```python
from build123d import *

# Parameters (mm, degrees)
F0_R     = 5
F1_DEPTH = 10
F2_DEPTH = 30


with BuildPart() as f1:
    # F0 (on Front) → F1 (new body, symmetric)
    with BuildSketch(Plane.XZ):
        with BuildLine():
            Line((-25, -43.3012701892), (-5, -8.6602540378))
            ThreePointArc((-5, -8.6602540378), (-5, 8.6602540378), (10, 0))
            ThreePointArc((10, 0), (8.6602540378, -5), (5, -8.6602540378))
            Line((5, -8.6602540378), (25, -43.3012701892))
            Line((25, -43.3012701892), (10, 100))
            ThreePointArc((10, 100), (0, 90), (-10, 100))
            Line((-10, 100), (-25, -43.3012701892))
        make_face()
        with BuildLine():
            Line((47.5, -82.2724133595), (45, -77.9422863406))
            ThreePointArc((45, -77.9422863406), (41.3397459622, -81.6025403784), (40, -86.6025403784))
            Line((40, -86.6025403784), (45, -86.6025403784))
            ThreePointArc((45, -86.6025403784), (45.6698729811, -84.1025403784), (47.5, -82.2724133595))
        make_face()
        with BuildLine():
            Line((-5, -8.6602540378), (-2.5, -4.3301270189))
            ThreePointArc((-2.5, -4.3301270189), (-2.5, 4.3301270189), (5, 0))
            ThreePointArc((5, 0), (4.3301270189, -2.5), (2.5, -4.3301270189))
            Line((2.5, -4.3301270189), (5, -8.6602540378))
            ThreePointArc((5, -8.6602540378), (8.6602540378, -5), (10, 0))
            ThreePointArc((10, 0), (-5, 8.6602540378), (-5, -8.6602540378))
        make_face()
        with BuildLine():
            Line((-45, -77.9422863406), (-25, -43.3012701892))
            Line((-25, -43.3012701892), (-57.4852813742, -79.9715100853))
            ThreePointArc((-57.4852813742, -79.9715100853), (-51.6042422288, -76.7320587858), (-45, -77.9422863406))
        make_face()
        with BuildLine():
            ThreePointArc((57.4852813742, -79.9715100853), (51.6042422288, -76.7320587858), (45, -77.9422863406))
            Line((45, -77.9422863406), (47.5, -82.2724133595))
            ThreePointArc((47.5, -82.2724133595), (52.5, -82.2724133595), (55, -86.6025403784))
            ThreePointArc((55, -86.6025403784), (50, -91.6025403784), (45, -86.6025403784))
            Line((45, -86.6025403784), (40, -86.6025403784))
            ThreePointArc((40, -86.6025403784), (42.2540333076, -92.9270956988), (48, -96.4004993496))
            ThreePointArc((48, -96.4004993496), (56.3245553203, -94.3485070709), (60, -86.6025403784))
            ThreePointArc((60, -86.6025403784), (59.3502089213, -83.0566141061), (57.4852813742, -79.9715100853))
        make_face()
        with BuildLine():
            ThreePointArc((-40, -86.6025403784), (-41.3397459622, -81.6025403784), (-45, -77.9422863406))
            Line((-45, -77.9422863406), (-47.5, -82.2724133595))
            ThreePointArc((-47.5, -82.2724133595), (-45.6698729811, -84.1025403784), (-45, -86.6025403784))
            Line((-45, -86.6025403784), (-40, -86.6025403784))
        make_face()
        with BuildLine():
            Line((0, -86.6025403784), (-40, -86.6025403784))
            ThreePointArc((-40, -86.6025403784), (-42.2540333076, -92.9270956988), (-48, -96.4004993496))
            Line((-48, -96.4004993496), (0, -86.6025403784))
        make_face()
        with BuildLine():
            ThreePointArc((48, -96.4004993496), (42.2540333076, -92.9270956988), (40, -86.6025403784))
            Line((40, -86.6025403784), (0, -86.6025403784))
            Line((0, -86.6025403784), (48, -96.4004993496))
        make_face()
        with BuildLine():
            Line((57.4852813742, -79.9715100853), (25, -43.3012701892))
            Line((25, -43.3012701892), (45, -77.9422863406))
            ThreePointArc((45, -77.9422863406), (51.6042422288, -76.7320587858), (57.4852813742, -79.9715100853))
        make_face()
        with BuildLine():
            ThreePointArc((10, 100), (0, 110), (-10, 100))
            ThreePointArc((-10, 100), (0, 90), (10, 100))
        make_face()
        with Locations((0, 100)):
            Circle(F0_R, mode=Mode.SUBTRACT)
        with BuildLine():
            Line((-47.5, -82.2724133595), (-45, -77.9422863406))
            ThreePointArc((-45, -77.9422863406), (-51.6042422288, -76.7320587858), (-57.4852813742, -79.9715100853))
            ThreePointArc((-57.4852813742, -79.9715100853), (-58.6602540378, -91.6025403784), (-48, -96.4004993496))
            ThreePointArc((-48, -96.4004993496), (-42.2540333076, -92.9270956988), (-40, -86.6025403784))
            Line((-40, -86.6025403784), (-45, -86.6025403784))
            ThreePointArc((-45, -86.6025403784), (-54.3301270189, -89.1025403784), (-47.5, -82.2724133595))
        make_face()
        with BuildLine():
            ThreePointArc((5, -8.6602540378), (0, -10), (-5, -8.6602540378))
            Line((-5, -8.6602540378), (-25, -43.3012701892))
            Line((-25, -43.3012701892), (-45, -77.9422863406))
            ThreePointArc((-45, -77.9422863406), (-41.3397459622, -81.6025403784), (-40, -86.6025403784))
            Line((-40, -86.6025403784), (0, -86.6025403784))
            Line((0, -86.6025403784), (40, -86.6025403784))
            ThreePointArc((40, -86.6025403784), (41.3397459622, -81.6025403784), (45, -77.9422863406))
            Line((45, -77.9422863406), (25, -43.3012701892))
            Line((25, -43.3012701892), (5, -8.6602540378))
        make_face()
        with BuildLine():
            ThreePointArc((2.5, -4.3301270189), (0, -5), (-2.5, -4.3301270189))
            Line((-2.5, -4.3301270189), (-5, -8.6602540378))
            ThreePointArc((-5, -8.6602540378), (0, -10), (5, -8.6602540378))
            Line((5, -8.6602540378), (2.5, -4.3301270189))
        make_face()
    extrude(amount=F1_DEPTH, both=True)

    # F0 (on Front) → F2 (join, symmetric)
    with BuildSketch(Plane.XZ):
        with Locations((0, 100)):
            Circle(F0_R)
        with BuildLine():
            Line((-2.5, -4.3301270189), (0, 0))
            Line((0, 0), (2.5, -4.3301270189))
            ThreePointArc((2.5, -4.3301270189), (4.3301270189, -2.5), (5, 0))
            ThreePointArc((5, 0), (-2.5, 4.3301270189), (-2.5, -4.3301270189))
        make_face()
        with BuildLine():
            Line((2.5, -4.3301270189), (0, 0))
            Line((0, 0), (-2.5, -4.3301270189))
            ThreePointArc((-2.5, -4.3301270189), (0, -5), (2.5, -4.3301270189))
        make_face()
        with BuildLine():
            ThreePointArc((-45, -86.6025403784), (-45.6698729811, -84.1025403784), (-47.5, -82.2724133595))
            Line((-47.5, -82.2724133595), (-50, -86.6025403784))
            Line((-50, -86.6025403784), (-45, -86.6025403784))
        make_face()
        with BuildLine():
            Line((-50, -86.6025403784), (-47.5, -82.2724133595))
            ThreePointArc((-47.5, -82.2724133595), (-54.3301270189, -89.1025403784), (-45, -86.6025403784))
            Line((-45, -86.6025403784), (-50, -86.6025403784))
        make_face()
        with BuildLine():
            Line((50, -86.6025403784), (47.5, -82.2724133595))
            ThreePointArc((47.5, -82.2724133595), (45.6698729811, -84.1025403784), (45, -86.6025403784))
            Line((45, -86.6025403784), (50, -86.6025403784))
        make_face()
        with BuildLine():
            ThreePointArc((55, -86.6025403784), (52.5, -82.2724133595), (47.5, -82.2724133595))
            Line((47.5, -82.2724133595), (50, -86.6025403784))
            Line((50, -86.6025403784), (45, -86.6025403784))
            ThreePointArc((45, -86.6025403784), (50, -91.6025403784), (55, -86.6025403784))
        make_face()
    extrude(amount=F2_DEPTH, both=True)


solid = f1.part
```
Could you check a few things on this model? Use its own coordinates, in mm. A direction names the side the tool comes from. Coordinates: 2 decimals unless noted, no trailing zeros. Write each loop counter-clockwise with the first axis right and the second up, starting at its lowest first coordinate (ties: lowest second). Pieces come first, ordered by that corner, then holes. Notation, with made-up numbers: (-16, -15) -> (20, -15) arc R13 cw to (20, -1) -> close; hole circle Ø6 at (-8.5, 25.5). An arc over 180 degrees is marked (long way). Write item = value, one per line. Start each with the question number.
(1) I want a section at D-D (z = 58). Please give me the cut outline in (x, y).
(2) Which directions (+Z, -Z, +X, -X, +Y, -Y) give clear straight access to the entire face, cutting with the end or side of a thin tool? Please do faces 4 (the face through (-54.995, 20.14, -86.383)), 5 (the face through (0, 30, 100)), 6 (the face through (-1, -10, -38)), 7 (the face through (23.664, -0.14, -91.433)), 8 (the face through (50, -30, -87)).
(3) I want a section at C-C (y = 4). Please give me the cut outline in (x, z).
(4) I want a section at B-B (x = -50). Please give me the cut outline in (y, z), plus the area to 3 significant figures.
(5) Will these pins go through, and if not, where does the flat tip stop? pin 1 (3 mm diameter, centred on x = 4, y = -24, fed in from +Z); pin 2 (10 mm diameter, centred on x = 8, z = 83.5, fed in from +Y); pin 3 (1.5 mm diameter, centred on y = -8.5, z = 71, fed in from +X).
(6) I need wall thicknesses on line 1 (Y direction, x = -9, z = 14); line 2 (Z direction, x = 3.5, y = -9); line 3 (X direction, y = 6, z = -73). Which ranges of each line are inside material? Lowest first, please. Write a range as [from, to].
(7) I want a section at A-A (y = 24). Please give me the cut outline in (x, z), plus the area to 3 significant figures.
(8) We'd pull the mould along X, two halves only. Please class faces 1 (the face through (17.605, -0.14, 27.346)), 2 (the face through (-24.34, -0.14, -91.57)), 3 (the face through (-1.08, 19.86, 95.12)): released by +X, released by -X, zero draft, split by the parting line, or undercut.
Result set:
q1.outline = (-14.4, -10) -> (14.4, -10) -> (14.4, 10) -> (-14.4, 10) -> close
q2.face_4 = +Y
q2.face_5 = +Z, -Z, +X, -X, +Y
q2.face_6 = -Y
q2.face_7 = -Z, +Y, -Y
q2.face_8 = +Z, -Z, +X, -X, -Y
q3.outline = (-57.49, -79.97) arc R10 ccw to (-48, -96.4) -> (0, -86.6) -> (48, -96.4) arc R10 ccw to (57.49, -79.97) -> (25, -43.3) -> (10, 100) arc R10 ccw to (-10, 100) -> (-25, -43.3) -> close
q4.outline = (-30, -91.6) -> (-10, -91.6) -> (-10, -96.6) -> (10, -96.6) -> (10, -91.6) -> (30, -91.6) -> (30, -81.6) -> (10, -81.6) -> (10, -71.52) -> (-10, -71.52) -> (-10, -81.6) -> (-30, -81.6) -> close
q4.area = 902 mm2
q5.pin_1 = 104.33
q5.pin_2 = 10
q5.pin_3 = 13.11
q6.line_1 = [-10, 10]
q6.line_2 = [-87.32, 109.37]
q6.line_3 = [-51.31, 51.31]
q7.outline = circle Ø10 at (-50, -86.6); circle Ø10 at (0, 0); circle Ø10 at (0, 100); circle Ø10 at (50, -86.6)
q7.area = 314 mm2
q8.face_1 = released by +X
q8.face_2 = undercut
q8.face_3 = split by the parting line
